Could you check a few things on this model? Use its own coordinates, in mm. Face numbers are marked on the shaded views. A direction names the side the tool comes from. Coordinates: 2 decimals unless noted, no trailing zeros. Loops run counter-clockwise (first coordinate to the right, second up) from the corner with the lowest first, then second, coordinate; pieces in that order, holes last.
from build123d import *

# Parameters (mm, degrees)
BOSS_EXTRUDE1_DEPTH   = 30
SKETCH2_R             = 1.75
CUT_EXTRUDE1_DEPTH    = 10
SKETCH3_R             = 1.9
BOSS_EXTRUDE2_DEPTH   = 155
BOSS_EXTRUDE2_2_DEPTH = 155
BOSS_EXTRUDE3_DEPTH   = 10
BOSS_EXTRUDE4_START   = -2
SKETCH6_R             = 2.9
SKETCH6_R_2           = 1.9
BOSS_EXTRUDE4_DEPTH   = 2
SKETCH7_W             = 11
SKETCH7_H             = 13
CUT_EXTRUDE2_DEPTH    = 240.426397876


with BuildPart() as part:
    # Sketch1 → Boss-Extrude1 (new body)
    with BuildSketch(Plane.XY):
        Polygon((30, 0), (0, 0), (0, 100), (180, 100), (180, 0), (150, 0), (150, 5), (175, 5), (175, 95), (5, 95), (5, 5), (30, 5), align=None)
    extrude(amount=-BOSS_EXTRUDE1_DEPTH)

    # Sketch2 → Cut-Extrude1 (cut)
    with BuildSketch(Plane.XZ):
        with Locations((15, -15)):
            Circle(SKETCH2_R)
        with Locations(Location((165, -15, 0), (0, 0, 90))):
            Circle(SKETCH2_R)
    extrude(amount=-CUT_EXTRUDE1_DEPTH, mode=Mode.SUBTRACT)



with BuildPart() as body_2:
    # Sketch3 → Boss-Extrude2 (new body)
    with BuildSketch(Plane.XZ.offset(-95)):
        with Locations((54.85, 5)):
            Circle(SKETCH3_R)
    extrude(amount=BOSS_EXTRUDE2_DEPTH)


with BuildPart() as body_3:
    # Sketch3 → Boss-Extrude2 2 (new body)
    with BuildSketch(Plane.XZ.offset(-95)):
        with Locations(Location((125.15, 5, 0), (0, 0, 180))):
            Circle(SKETCH3_R)
    extrude(amount=BOSS_EXTRUDE2_2_DEPTH)


with BuildPart() as part_1:
    add(part.part)

    add(body_2.part)  # Boss-Extrude3 merges body 2

    add(body_3.part)  # Boss-Extrude3 merges body 3
    # Sketch5 → Boss-Extrude3 (add)
    with BuildSketch(Plane.XY):
        Polygon((0, 95), (5, 95), (175, 95), (180, 95), (180, 100), (0, 100), align=None)
    extrude(amount=BOSS_EXTRUDE3_DEPTH)

    # Sketch6 → Boss-Extrude4 (add)
    # profile 1 of 2: a face of its own
    with BuildSketch(Plane.XZ.offset(60).offset(BOSS_EXTRUDE4_START)):
        with Locations((54.85, 5)):
            Circle(SKETCH6_R)
        with Locations((54.85, 5)):
            Circle(SKETCH6_R_2, mode=Mode.SUBTRACT)
    # profile 2 of 2: a face of its own
    with BuildSketch(Plane.XZ.offset(60).offset(BOSS_EXTRUDE4_START)):
        with Locations((125.15, 5)):
            Circle(SKETCH6_R)
        with Locations(Location((125.15, 5, 0), (0, 0, 180))):
            Circle(SKETCH6_R_2, mode=Mode.SUBTRACT)
    extrude(amount=BOSS_EXTRUDE4_DEPTH)

    # Sketch7 → Cut-Extrude2 (cut, through all)
    with BuildSketch(Plane.XZ.offset(-95)):
        with Locations((89.880118622, 0.075917746)):
            Rectangle(SKETCH7_W, SKETCH7_H)
    extrude(amount=-CUT_EXTRUDE2_DEPTH, mode=Mode.SUBTRACT)


solid = part_1.part
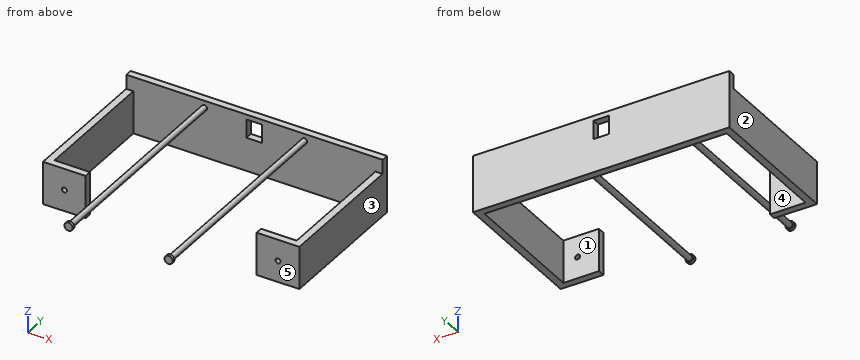
(1) Imagine slicing it at A-A, the plane y = 16. Write out the boundary of the cut face in (x, z).
Answers:
outline: (0, -30) - (5, -30) - (5, 0) - (0, 0) - close; circle Ø3.8 at (54.85, 5); circle Ø3.8 at (125.15, 5); (175, -30) - (180, -30) - (180, 0) - (175, 0) - close
(2) Imagine slicing it at C-C, the plane y = -29.5. Write out the boundary of the cut face in (x, z), and give its area (3 significant figures).
Answers:
outline: circle Ø3.8 at (54.85, 5); circle Ø3.8 at (125.15, 5)
area: 22.7 mm2
(3) I need wall thicknesses on probe 1 along X at (y, z) = (56.5, -28); probe 2 along Y at (x, z) = (151, -9); probe 3 along Z at (x, y) = (165, 3.5). Which ranges of each line are inside material? Lowest first, please.
Answers:
probe 1: x = 0 to 5, 175 to 180
probe 2: y = 0 to 5, 95 to 100
probe 3: z = -30 to -16.75, -13.25 to 0
(4) For pin 1 (2 mm diameter, centred on x = 106, z = -5, fed in from -Y); pin 2 (24 mm diameter, centred on x = 159.5, z = -11.5, fed in from -Y); pin 3 (1.5 mm diameter, centred on y = -41.5, z = 1, fed in from -X), each with a flat end and sliding along its axis, tell me the tip position at first contact or that it passes through.
Answers:
pin 1: stops at y = 95
pin 2: stops at y = 0
pin 3: passes through
(5) Imagine slicing it at B-B, the plane z = -24. Write out the boundary of the cut face in (x, y), and give its area (3 significant figures).
Answers:
outline: (0, 0) - (30, 0) - (30, 5) - (5, 5) - (5, 95) - (175, 95) - (175, 5) - (150, 5) - (150, 0) - (180, 0) - (180, 100) - (0, 100) - close
area: 2,100 mm2
(6) We'd pull the mould along X, two halves only. Please class the marked faces 3, 4 and 5: +X half, -X half, draft (parallel to the pull), parting line (faces both ways), or undercut.
Answers:
face 3: +X half
face 4: undercut
face 5: draft
(7) Which directions (+Z, -Z, +X, -X, +Y, -Y) give clear straight access to the entire face, cutting with the end or side of a thin tool? Please do the marked faces 1 and 2.
Answers:
face 1: +Z, -Z
face 2: +Z, -Z, -X, +Y, -Y
(8) Imagine slicing it at D-D, the plane x = 147. Write out the boundary of the cut face in (y, z), and give its area (3 significant figures).
Answers:
outline: (95, -30) - (100, -30) - (100, 10) - (95, 10) - close
area: 200 mm2
